from build123d import *

# Parameters (mm, degrees)
F0_R     = 10
F1_DEPTH = 0.5
F2_DEPTH = 3
F3_R     = 10
F3_R_2   = 3
F4_DEPTH = 0.5
F5_R     = 10
F6_DEPTH = 0.5


with BuildPart() as f1:
    # F0 (on Top) → F1 (new body)
    with BuildSketch(Plane.XY):
        Circle(F0_R)
        with BuildLine():
            ThreePointArc((0, 3), (2.1213203436, 2.1213203436), (3, 0))
            ThreePointArc((3, 0), (2.1213203436, -2.1213203436), (0, -3))
            Line((0, -3), (-6, -3))
            ThreePointArc((-6, -3), (-9, 0), (-6, 3))
            Line((-6, 3), (0, 3))
        make_face(mode=Mode.SUBTRACT)
        with BuildLine():
            ThreePointArc((-6, -3), (-3.8786796564, -2.1213203436), (-3, 0))
            ThreePointArc((-3, 0), (-3.8786796564, 2.1213203436), (-6, 3))
            ThreePointArc((-6, 3), (-9, 0), (-6, -3))
        make_face()
        with BuildLine():
            ThreePointArc((-3, 0), (-2.1213203436, 2.1213203436), (0, 3))
            Line((0, 3), (-6, 3))
            ThreePointArc((-6, 3), (-3.8786796564, 2.1213203436), (-3, 0))
        make_face()
        with BuildLine():
            Line((-6, -3), (0, -3))
            ThreePointArc((0, -3), (-2.1213203436, -2.1213203436), (-3, 0))
            ThreePointArc((-3, 0), (-3.8786796564, -2.1213203436), (-6, -3))
        make_face()
        with BuildLine():
            ThreePointArc((0, -3), (2.1213203436, -2.1213203436), (3, 0))
            ThreePointArc((3, 0), (2.1213203436, 2.1213203436), (0, 3))
            ThreePointArc((0, 3), (-2.1213203436, 2.1213203436), (-3, 0))
            ThreePointArc((-3, 0), (-2.1213203436, -2.1213203436), (0, -3))
        make_face()
    extrude(amount=F1_DEPTH)

    # F0 (on Top) → F2 (join)
    with BuildSketch(Plane.XY):
        Circle(F0_R)
        with BuildLine():
            ThreePointArc((0, 3), (2.1213203436, 2.1213203436), (3, 0))
            ThreePointArc((3, 0), (2.1213203436, -2.1213203436), (0, -3))
            Line((0, -3), (-6, -3))
            ThreePointArc((-6, -3), (-9, 0), (-6, 3))
            Line((-6, 3), (0, 3))
        make_face(mode=Mode.SUBTRACT)
    extrude(amount=F2_DEPTH)

    # F3 (on face) → F4 (join)
    with BuildSketch(Plane.XY.offset(3)):
        Circle(F3_R)
        with Locations((-6, 0)):
            Circle(F3_R_2, mode=Mode.SUBTRACT)
    extrude(amount=F4_DEPTH)

    # F5 (on face) → F6 (join)
    with BuildSketch(Plane.XY.offset(3.5)):
        Circle(F5_R)
    extrude(amount=F6_DEPTH)


solid = f1.part
Geometry check sheet. Reference: the model listing, model coordinates, mm. A direction names the side the tool comes from. Coordinates: 2 decimals unless noted, no trailing zeros. Write each loop counter-clockwise with the first axis right and the second up, starting at its lowest first coordinate (ties: lowest second). Pieces come first, ordered by that corner, then holes. Notation, with made-up numbers: (49, 5) -> (87, 5) arc R11 cw to (87, 10) -> close; hole circle Ø7 at (7, 38.25). An arc over 180 degrees is marked (long way). One line per question, with ' | ' between items.
1. Cross-section at A-A on z = 1.9. Record the cut outline in (x, y), and give its area (3 significant figures).
Answers:
outline: circle Ø20 at (0, 0); hole (-6, -3) -> (0, -3) arc R3 ccw to (0, 3) -> (-6, 3) arc R3 ccw to start | area: 250 mm²
2. Thickness scan on probe 1 along Z at (x, y) = (1.5, 0); probe 2 along X at (y, z) = (-1, 2.95); probe 3 along X at (y, z) = (0.5, 2). Record the ranges inside material, lowest first. Write a range as from..to.
Answers:
probe 1: z = 0..0.5, 3..4 | probe 2: x = -9.95..-8.83, 2.83..9.95 | probe 3: x = -9.99..-8.96, 2.96..9.99
3. Draft check along X on faces 1 (the flat face through (0, 0, 0)), 2 (the flat face through (-3, 3, 2)), 3 (the cylindrical face through (-2.17, -9.76, 1.97)). Enter one of: +X half, -X half, draft (parallel to the pull), parting line (faces both ways), or undercut.
Answers:
face 1: draft | face 2: undercut | face 3: parting line
4. Set-up check for faces 4 (the flat face through (0, 0, 4)), 5 (the flat face through (-1, 0, 3)): record each of +Z, -Z, +X, -X, +Y, -Y from which the full face is reachable in a straight line by a thin tool's end or side.
Answers:
face 4: +Z, +X, -X, +Y, -Y | face 5: none
5. Cross-section at B-B on x = -5. Record the cut outline in (y, z), and give its area (3 significant figures).
Answers:
outline: (-8.66, 0) -> (8.66, 0) -> (8.66, 4) -> (-8.66, 4) -> close; hole (-3, 0.5) -> (3, 0.5) -> (3, 3) -> (2.83, 3) -> (2.83, 3.5) -> (-2.83, 3.5) -> (-2.83, 3) -> (-3, 3) -> close | area: 51.5 mm²
6. Depth check by flat-ended pin: pin 1 Ø1.5 at (y, z) = (-2, 3.5) entering from +X; pin 2 Ø0.8 at (x, z) = (-3.5, 2) entering from -Y. Enter the tip coordinate at first touch or a pass-through.
Answers:
pin 1: stops at x = 9.92 | pin 2: stops at y = -9.51
7. Cross-section at C-C on y = 0.75. Record the cut outline in (x, z).
Answers:
outline: (-9.97, 0) -> (9.97, 0) -> (9.97, 4) -> (-9.97, 4) -> close; hole (-8.9, 0.5) -> (2.9, 0.5) -> (2.9, 3) -> (-3.1, 3) -> (-3.1, 3.5) -> (-8.9, 3.5) -> close
8. Cross-section at D-D on x = -1.25. Record the cut outline in (y, z), and give its area (3 significant figures).
Answers:
outline: (-9.92, 0) -> (9.92, 0) -> (9.92, 4) -> (-9.92, 4) -> close; hole (-3, 0.5) -> (3, 0.5) -> (3, 3) -> (-3, 3) -> close | area: 64.4 mm²
